Model file for the job. Use its own axes, mm. Give positions to 0.01 mm unless a question says otherwise; leave off trailing zeros. Order: outer loops, then holes, each group sorted by start corner. A loop starts at its lowest first (then second) coordinate and runs counter-clockwise, first axis right, second up. Notation, with made-up numbers: (51, -19) - (90, -19) arc R22 cw to (90, 19) - close; hole circle Ø5 at (39, 22). An arc over 180 degrees is marked (long way). Return JSON: item names as keys, results as strings. Group by question number.
from build123d import *


with BuildPart() as f1:
    # F0 (on Front) → F1 (revolve)
    with BuildSketch(Plane.XZ):
        with BuildLine():
            Line((-170.656085, -914.4), (0, -914.4))
            Line((0, -914.4), (0, 914.4))
            ThreePointArc((0, 914.4), (-133.642487, 808.103429), (-60.143852, 653.969636))
            Line((-60.143852, 653.969636), (-60.418386, 632.761954))
            Line((-60.418386, 632.761954), (-171.262137, 634.196832))
            ThreePointArc((-171.262137, 634.196832), (-214.594867, 616.90151), (-233.006095, 574.031004))
            Line((-233.006095, 574.031004), (-239.706635, 56.417))
            Line((-239.706635, 56.417), (-158.82012, -0.076605))
            Line((-158.82012, -0.076605), (-170.656085, -914.4))
        make_face()
    revolve(axis=Axis((0, 0, 0), (0, 0, -1)))


solid = f1.part
(1) Slice it at B-B (z = 30). Give the cut face in (x, y), and give its area (3 significant figures).
(2) Slice it at A-A (z = 711.5). Give the cut face in (x, y), and give its area (3 significant figures).
(3) Drop flat-ended pins along their axis: pin 1 Ø12 at (x, z) = (-137, -492.5) entering from -Y; pin 2 Ø6 at (y, z) = (-112.5, -423) entering from -X; pin 3 Ø6 at (x, z) = (-99.5, 24) entering from -Y. Give the stop position or say it passes through.
(4) Drill centre lines: L1, parallel to Z at x = 7, y = 154.5; L2, parallel to Z at x = -13, y = -93.5; L3, parallel to Z at x = 27.5, y = -147. Where is each one in solid material? Low to high.
(5) Pull direction Z, two halves, no side cores. Call faces 1 (the face through (35.73, -160.9, -463.64)), 2 (the face through (51.25, -230.78, 311.6)), 3 (the face through (2, 2, -914.4)): released by +Z, released by -Z, zero draft, split by the parting line, or undercut.
Result set:
{
 "1": {"outline": "circle Ø403.77 at (0, 0)", "area": "128,000 mm²"},
 "2": {"outline": "circle Ø240.76 at (0, 0)", "area": "45,500 mm²"},
 "3": {"pin 1": "stops at y = -100.64", "pin 2": "stops at x = -122.49", "pin 3": "stops at y = -171"},
 "4": {"L1": "z = -914.4 to 633.98", "L2": "z = -914.4 to 633.2, 677.73 to 876.75", "L3": "z = -914.4 to 633.92"},
 "5": {"face 1": "undercut", "face 2": "released by +Z", "face 3": "released by -Z"}
}
